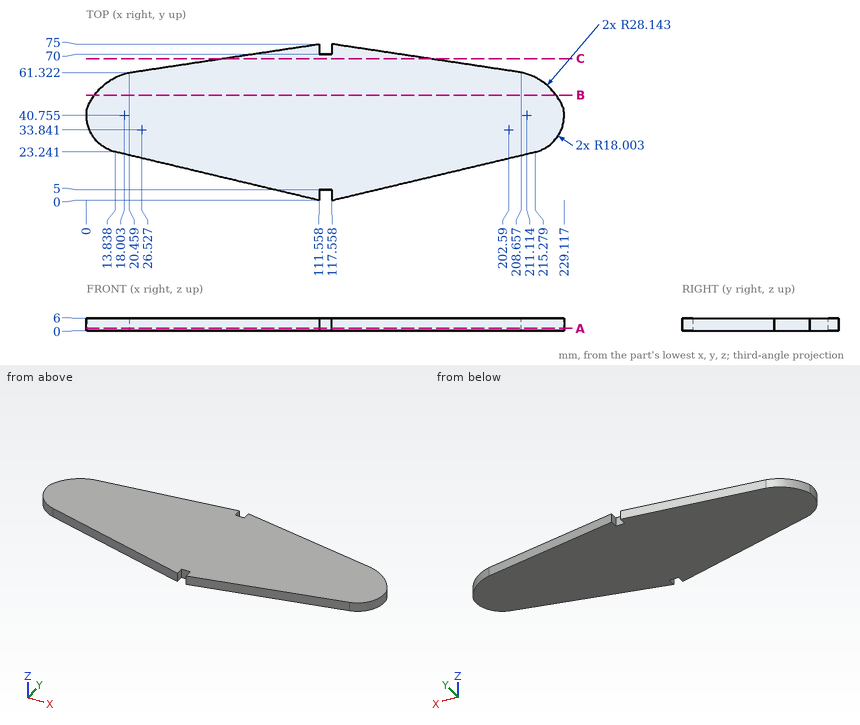
Source: three-view drawing plus pictorial views. Frame: mm from the lowest corner of the part. Round coordinates to 2 decimals unless told otherwise and drop trailing zeros. Loops run counter-clockwise (first coordinate to the right, second up) from the corner with the lowest first, then second, coordinate; pieces in that order, holes last.
1. Ray query, L1, parallel to X at y = 26, z = 4.75 (1 decimal); L2, parallel to X at y = 44, z = 3.25 (1 decimal); L3, parallel to Y at x = 126, z = 4. Return the intervals inside material, ascending.
2. Section query C-C on y = 68. Output: boundary loops of the cut face in (x, z) (1 decimal).
3. Section query B-B on y = 50.5. Output: boundary loops of the cut face in (x, z).
4. Contact query for flat-ended pins moving along their axis: pin 1 (2 mm diameter, centred on x = 97.5, z = 3.5, fed in from -Y) (1 decimal); pin 2 (1.8 mm diameter, centred on x = 114, z = 4.5, fed in from -Y); pin 3 (1.5 mm diameter, centred on y = 26, z = 5, fed in from -X). Output: stop coordinate, or through.
5. Section query A-A on z = 1.25. Output: boundary loops of the cut face in (x, y) (1 decimal).
Answers below:
1. L1: x = 7.7 to 221.4
1. L2: x = 0.3 to 228.8
1. L3: y = 2.01 to 73.73
2. outline: (64.9, 0) - (164.2, 0) - (164.2, 6) - (64.9, 6) - close
3. outline: (3.84, 0) - (225.27, 0) - (225.27, 6) - (3.84, 6) - close
4. pin 1: stops at y = 3.1
4. pin 2: stops at y = 5
4. pin 3: stops at x = 6.69
5. outline: (0.3, 44.1) arc R18 ccw to (13.8, 23.2) - (111.6, 0) - (111.6, 5) - (117.6, 5) - (117.6, 0) - (215.3, 23.2) arc R18 ccw to (228.8, 44.1) arc R28.1 ccw to (208.7, 61.3) - (117.6, 75) - (117.6, 70) - (111.6, 70) - (111.6, 75) - (20.5, 61.3) arc R28.1 ccw to start
